```python
from build123d import *

# Parameters (mm, degrees)
BOSS_EXTRUDE1_DEPTH            = 800
SHELL1_T                       = -1.5
M4_CLEARANCE_HOLE1_D           = 4.5
M4_CLEARANCE_HOLE1_CSINK_D     = 4.55
M4_CLEARANCE_HOLE1_CSINK_ANGLE = 100


with BuildPart() as part:
    # Sketch1 → Boss-Extrude1 (new body)
    with BuildSketch(Plane(origin=(0, 0, 0), x_dir=(1, 0, 0), z_dir=(0, 1, 0))):
        with BuildLine():
            Line((-140, 0), (140, 0))
            ThreePointArc((140, 0), (0, 140), (-140, 0))
        make_face()
    extrude(amount=BOSS_EXTRUDE1_DEPTH)

    # Shell1
    shell1_openings = [part.faces().sort_by_distance(p)[0] for p in [
        (0, 400, 0),
    ]]
    offset(amount=SHELL1_T, openings=shell1_openings)

    # M4 Clearance Hole1 (through all)
    with Locations(Plane(origin=(0, 800, 0), x_dir=(1, 0, 0), z_dir=(0, 1, 0))):
        with Locations((-130, 5), (-115, 5)):
            CounterSinkHole(M4_CLEARANCE_HOLE1_D / 2, M4_CLEARANCE_HOLE1_CSINK_D / 2, counter_sink_angle=M4_CLEARANCE_HOLE1_CSINK_ANGLE)


solid = part.part
```
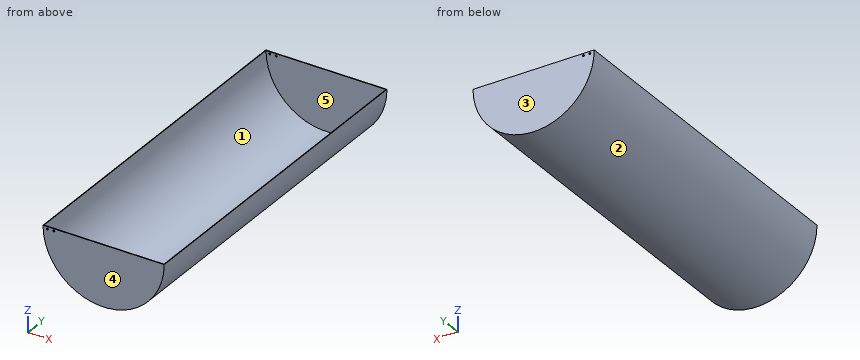
Geometry: final body of the model. Coordinates: model frame, mm. Face numbers are marked on the shaded views. A direction names the side the tool comes from. Coordinates: 2 decimals unless noted, no trailing zeros. Order: outer loops, then holes, each group sorted by start corner. A loop starts at its lowest first (then second) coordinate and runs counter-clockwise, first axis right, second up. Notation, with made-up numbers: M 25.5,18 L 56.5,18 A23 cw 56.5,30 Z; hole C 19,-26 d6. An arc over 180 degrees is marked long. Answer in a Markdown table with one row per item. Add a question column.
Q1. Mould query, pull axis Y, two halves, no side actions, for the marked faces 3, 4 and 5. Classes: released by +Y, released by -Y, zero draft, split by the parting line, or undercut.
Q2. Section query B-B on x = -79. Return the cut outline in (y, z), and give its area (3 significant figures).
Q3. Reachability of the marked faces 1 and 2 from +Z, -Z, +X, -X, +Y, -Y: full face, straight path, thin tool, end or side. Return the list, or none.
Q4. Section query A-A on z = -76. Return the cut outline in (x, y), and give its area (3 significant figures).
Q5. Section query D-D on y = 581. Return the cut outline in (x, z), and give its area (3 significant figures).
Q6. Contact query for flat-ended pins moving along their axis: P1, Ø2, axis at x = 17, y = 634, coming from the +Z side; P2, Ø2, axis at x = -103, y = 620.5, coming from the -Z side; P3, Ø10, axis at x = 4.5, y = 218, coming from the +Z side. Output: stop coordinate, or through.
Q7. Section query C-C on z = -119. Return the cut outline in (x, y).
Q8. Line query: L1, parallel to Y at x = -8, z = -18; L2, parallel to X at y = 248.5, z = -80; L3, parallel to Z at x = 6.5, y = 690. Output: solid intervals per line, ascending.
Completed:
| question | item | result |
|---|---|---|
| 1 | face 3 | released by +Y |
| 1 | face 4 | released by -Y |
| 1 | face 5 | undercut |
| 2 | outline | M 0,-115.58 L 800,-115.58 L 800,0 L 798.5,0 L 798.5,-113.76 L 1.5,-113.76 L 1.5,0 L 0,0 Z |
| 2 | area | 1,800 mm2 |
| 3 | face 1 | +Z |
| 3 | face 2 | -Z, +Y, -Y |
| 4 | outline | M -117.58,0 L 117.58,0 L 117.58,800 L -117.58,800 Z; hole M -115.79,1.5 L 115.79,1.5 L 115.79,798.5 L -115.79,798.5 Z |
| 4 | area | 3,560 mm2 |
| 5 | outline | M -140,0 A140 ccw 140,0 L 138.5,0 A138.5 cw -138.5,0 Z |
| 5 | area | 656 mm2 |
| 6 | P1 | stops at z = -137.33 |
| 6 | P2 | stops at z = -95.9 |
| 6 | P3 | stops at z = -138.17 |
| 7 | outline | M -73.75,0 L 73.75,0 L 73.75,800 L -73.75,800 Z; hole M -70.86,1.5 L 70.86,1.5 L 70.86,798.5 L -70.86,798.5 Z |
| 8 | L1 | y = 0 to 1.5, 798.5 to 800 |
| 8 | L2 | x = -114.89 to -113.06, 113.06 to 114.89 |
| 8 | L3 | z = -139.85 to -138.35 |
